CAD build for the part. Positions are in the model's coordinates, mm. A direction names the side the tool comes from. Round coordinates to 2 decimals unless told otherwise and drop trailing zeros. Order: outer loops, then holes, each group sorted by start corner. A loop starts at its lowest first (then second) coordinate and runs counter-clockwise, first axis right, second up. Notation, with made-up numbers: (71, 28.5) - (76, 28.5) arc R22 cw to (76, 36.5) - close; hole circle Ø6 at (65, 9.5). An arc over 180 degrees is marked (long way). Use one line per item in the form item = value. Start each with the question number.
from build123d import *


with BuildPart() as part:
    # Sketch1 → Revolve: OD (revolve)
    with BuildSketch(Plane.XY):
        with BuildLine():
            Line((0, 12.065), (0.9525, 12.065))
            Line((0.9525, 12.065), (0.9525, 11.43))
            Line((0.9525, 11.43), (1.524, 11.43))
            ThreePointArc((1.524, 11.43), (1.849213675, 11.54774359), (2.023672131, 11.846393443))
            ThreePointArc((2.023672131, 11.846393443), (2.286, 12.065), (2.548327869, 11.846393443))
            ThreePointArc((2.548327869, 11.846393443), (2.722786325, 11.54774359), (3.048, 11.43))
            Line((3.048, 11.43), (5.842, 11.43))
            ThreePointArc((5.842, 11.43), (6.201210245, 11.578789755), (6.35, 11.938))
            Line((6.35, 11.938), (6.35, 12.065))
            Line((6.35, 12.065), (7.120204895, 12.065))
            Line((7.120204895, 12.065), (11.353409628, 0.434365582))
            ThreePointArc((11.353409628, 0.434365582), (11.410705846, 0.220533186), (11.43, 0))
            Line((11.43, 0), (0, 0))
            Line((0, 0), (0, 12.065))
        make_face()
    revolve(axis=Axis((-0.699583002, 0, 0), (1, 0, 0)))

    # Sketch3 → Cut-Revolve: ID (revolve, cut)
    with BuildSketch(Plane.XY):
        Polygon((0, 0), (0, 7.62), (2.0955, 7.62), (2.0955, 11.303), (5.775743288, 11.303), (9.889698846, 0), align=None)
    revolve(axis=Axis((-1.469925142, 0, 0), (1, 0, 0)), mode=Mode.SUBTRACT)


solid = part.part
(1) Which spindle directions (+Z, -Z, +X, -X, +Y, -Y) get a long thin tool onto all of the face, cutting with end or side? Do faces 4 (the cylindrical face through (1.06, -1.65, -7.44)), 5 (the flat face through (2.095, -2.4, -7.4)), 6 (the cylindrical face through (0.48, 11.51, 3.62)). Say none if no direction does.
(2) Slice it at B-B (x = 9.5). Give the cut face in (y, z), and give its area (3 significant figures).
(3) Flat gauge pins, fed straight in: P1, Ø5, axis at y = -9.5, z = -5, coming from the +X side; P2, Ø1, axis at x = 6, z = -6.5, coming from the +Y side; P3, Ø3, axis at x = 2, z = 7.5, coming from the +Y side. Where does each tip first touch, or does it go through?
(4) Wall check: line 1 (Z direction, x = 1.5, y = 0); line 2 (Y direction, x = 4, z = -8); line 3 (Z direction, x = 2.75, y = -7). Give the ranges that are in metal, low to high. Write a range as [from, to].
(5) Slice it at A-A (x = 4.5). Give the cut face in (y, z), and give its area (3 significant figures).
(6) Mould opens along Y. For faces 1 (the flat face through (0.952, 11, -4)), 2 (the conical face through (11.148, -0.217, -0.975)), 3 (the conical face through (9.69, 0.52, 0.16)) say: pulls with the +Y half, pulls with the -Y half, needs draft (parallel to the pull), parting line crosses it, or undercut.
Results list:
q1.face_4 = -X
q1.face_5 = none
q1.face_6 = +X, -X
q2.outline = circle Ø11.05 at (0, 0); hole circle Ø2.14 at (0, 0)
q2.area = 92.4 mm²
q3.P1 = 8.51
q3.P2 = 10.38
q3.P3 = 10.45
q4.line_1 = [-11.43, -7.62], [7.62, 11.43]
q4.line_2 = [-8.16, -7.98], [7.98, 8.16]
q4.line_3 = [-9.16, -8.87], [8.87, 9.16]
q5.outline = circle Ø22.86 at (0, 0); hole circle Ø22.61 at (0, 0)
q5.area = 9.07 mm²
q6.face_1 = needs draft
q6.face_2 = parting line crosses it
q6.face_3 = undercut
